```python
from build123d import *

# Parameters (mm, degrees)
SKETCH1_R           = 205
SKETCH1_R_2         = 15
BOSS_EXTRUDE1_DEPTH = 20
CHAMFER1_SIZE       = 2


with BuildPart() as part:
    # Sketch1 → Boss-Extrude1 (new body)
    with BuildSketch(Plane.XY):
        Circle(SKETCH1_R)
        with Locations((0, 170)):
            Circle(SKETCH1_R_2, mode=Mode.SUBTRACT)
        with Locations((120.208152802, 120.208152802)):
            Circle(SKETCH1_R_2, mode=Mode.SUBTRACT)
        with Locations((170, 0)):
            Circle(SKETCH1_R_2, mode=Mode.SUBTRACT)
        with Locations((120.208152802, -120.208152802)):
            Circle(SKETCH1_R_2, mode=Mode.SUBTRACT)
        with Locations((0, -170)):
            Circle(SKETCH1_R_2, mode=Mode.SUBTRACT)
        with Locations((-120.208152802, -120.208152802)):
            Circle(SKETCH1_R_2, mode=Mode.SUBTRACT)
        with Locations((-170, 0)):
            Circle(SKETCH1_R_2, mode=Mode.SUBTRACT)
        with Locations((-120.208152802, 120.208152802)):
            Circle(SKETCH1_R_2, mode=Mode.SUBTRACT)
    extrude(amount=BOSS_EXTRUDE1_DEPTH)

    # Chamfer1
    chamfer1_edges = [part.edges().sort_by_distance(p)[0] for p in [
        (-205, 0, 0),
        (-205, 0, 20),
    ]]
    chamfer(chamfer1_edges, length=CHAMFER1_SIZE)


solid = part.part
```
Can you work these out from the model? Positions are in its coordinate system, mm. Give positions to 0.01 mm unless a question says otherwise; leave off trailing zeros. Order: outer loops, then holes, each group sorted by start corner. A loop starts at its lowest first (then second) coordinate and runs counter-clockwise, first axis right, second up. Notation, with made-up numbers: M -32,8 L 0,8 A14 cw 0,30 Z; hole C 2,16 d2. An arc over 180 degrees is marked long. Write item = value, one per line. Start each with the question number.
Q1. Will these pins go through, and if not, where does the flat tip stop? pin 1 Ø4 at (x, z) = (-90, 9.5) entering from -Y; pin 2 Ø12 at (x, z) = (82, 2.5) entering from +Y; pin 3 Ø12 at (x, z) = (128.5, 14) entering from -Y.
Q2. Suppose I cut it at A-A (y = 0). Write out the boundary of the cut face in (x, z), plus the area to 3 significant figures.
Q3. Suppose I cut it at C-C (z = 7.75). Count the separate pieces of the cut face and the enclosed holes in it, plus the area to 3 significant figures.
Q4. I need wall thicknesses on probe 1 along Y at (x, z) = (111.5, 15); probe 2 along X at (y, z) = (124, 10.75); probe 3 along Y at (x, z) = (-170, 11.5). Which ranges of each line are inside material? Lowest first, please. Write a range as [from, to].
Q5. We'd pull the mould along X, two halves only. Please class faces 1 (the flat face through (-3, 3, 0)), 2 (the cylindrical face through (116.956, 105.565, 9.86)), 3 (the cylindrical face through (-44.44, -200.125, 9.888)): pulls with the +X half, pulls with the -X half, needs draft (parallel to the pull), parting line crosses it, or undercut.
Check result:
q1.pin_1 = -185.15
q1.pin_2 = 190.39
q1.pin_3 = -164.37
q2.outline = M -205,2 L -203,0 L -185,0 L -185,20 L -203,20 L -205,18 Z; M -155,0 L 155,0 L 155,20 L -155,20 Z; M 185,0 L 203,0 L 205,2 L 205,18 L 203,20 L 185,20 Z
q2.area = 6,990 mm2
q3.separate_pieces = 1
q3.enclosed_holes = 8
q3.area = 126,000 mm2
q4.probe_1 = [-172.03, -132.42], [-107.99, 107.99], [132.42, 172.03]
q4.probe_2 = [-163.25, -134.72], [-105.7, 105.7], [134.72, 163.25]
q4.probe_3 = [-114.56, -15], [15, 114.56]
q5.face_1 = needs draft
q5.face_2 = undercut
q5.face_3 = parting line crosses it
